```python
from build123d import *

# Parameters (mm, degrees)
BOSS_EXTRUDE1_DEPTH = 1.5875
FILLET1_R           = 2.54
SKETCH6_OUTSIDE_W   = 130.286
SKETCH6_OUTSIDE_H   = 130.286
SKETCH6_OUTSIDE_W_2 = 99
SKETCH6_OUTSIDE_H_2 = 100
CUT_EXTRUDE2_DEPTH  = 71.728496069
SKETCH7_R           = 38.5
BOSS_EXTRUDE2_DEPTH = 0.1


with BuildPart() as part:
    # Sketch1 → Boss-Extrude1 (new body)
    with BuildSketch(Plane.XY):
        Polygon((40, 50), (-40, 50), (-40, 48), (-48, 48), (-48, 40), (-50, 40), (-50, -37.864895224), (-50, -40), (-48, -40), (-48, -48), (-40, -48), (-40, -50), (-37.864895224, -50), (40, -50), (40, -48), (48, -48), (48, -40), (50, -40), (50, 40), (48, 40), (48, 48), (40, 48), align=None)
    extrude(amount=BOSS_EXTRUDE1_DEPTH)

    # Fillet1
    # the kernel refuses this fillet: 2.54 mm, written as the material it adds along each edge
    with BuildSketch(Plane(origin=(-48, -40, 0), x_dir=(0, -1, 0), z_dir=(0, 0, 1)), Plane(origin=(40, -48, 0), x_dir=(1, 0, 0), z_dir=(0, 0, 1)), Plane(origin=(48, 40, 0), x_dir=(0, 1, 0), z_dir=(0, 0, 1)), Plane(origin=(-40, 48, 0), x_dir=(-1, 0, 0), z_dir=(0, 0, 1))) as fillet1_piece_1:
        with BuildLine():
            CenterArc((2.481934729, -2.54), FILLET1_R, 90, 77.725329785)
            Line((0, -2), (-0.049638695, -1.9892))
            ThreePointArc((-0.049638695, -1.9892), (-0.0508, -1), (-0.0508, 0))
            Line((-0.0508, 0), (0, 0.0508))
            Line((0, 0.0508), (2.481934729, 0.0508))
            Line((2.481934729, 0.0508), (2.481934729, 0))
        make_face()
    extrude(amount=1.5875)
    with BuildSketch(Plane(origin=(-40, -48, 0), x_dir=(-3.737454790095179e-12, -1.0, 0), z_dir=(0, 0, 1)), Plane(origin=(48, -40, 0), x_dir=(1.0, -3.7339020764163554e-12, 0), z_dir=(0, 0, 1)), Plane(origin=(-48, 40, 0), x_dir=(-1.0, 3.737454790095126e-12, 0), z_dir=(0, 0, 1))) as fillet1_piece_2:
        with BuildLine():
            CenterArc((2.54, -2.481934729), FILLET1_R, 102.274670215, 77.725329785)
            Line((0, -2.481934729), (-0.0508, -2.481934729))
            Line((-0.0508, -2.481934729), (-0.0508, 0))
            Line((-0.0508, 0), (0, 0.0508))
            ThreePointArc((0, 0.0508), (1, 0.0508), (1.9892, 0.049638695))
            Line((1.9892, 0.049638695), (2, 0))
        make_face()
    extrude(amount=1.5875)
    with BuildSketch(Plane(origin=(40, 48, 0), x_dir=(1, 0, 0), z_dir=(0, 0, 1))) as fillet1_piece_3:
        with BuildLine():
            CenterArc((2.481934729, 2.54), FILLET1_R, 192.274670215, 77.725329785)
            Line((0, 2), (-0.049638695, 1.9892))
            ThreePointArc((-0.049638695, 1.9892), (-0.0508, 1), (-0.0508, 0))
            Line((-0.0508, 0), (0, -0.0508))
            Line((0, -0.0508), (2.481934729, -0.0508))
            Line((2.481934729, -0.0508), (2.481934729, 0))
        make_face()
    extrude(amount=1.5875)

    # Sketch6 outside → Cut-Extrude2 (cut, through all)
    with BuildSketch(Plane.XY.offset(1.5875)):
        Rectangle(SKETCH6_OUTSIDE_W, SKETCH6_OUTSIDE_H)
        Rectangle(SKETCH6_OUTSIDE_W_2, SKETCH6_OUTSIDE_H_2, mode=Mode.SUBTRACT)
    extrude(amount=-CUT_EXTRUDE2_DEPTH, mode=Mode.SUBTRACT)

    # Sketch7 → Boss-Extrude2 (add)
    with BuildSketch(Plane(origin=(0, 0, 0), x_dir=(-1, 0, 0), z_dir=(0, 0, -1))):
        with Locations(Location((0, 0, 0), (0, 0, 180))):
            Circle(SKETCH7_R)
    extrude(amount=BOSS_EXTRUDE2_DEPTH)


solid = part.part
```
The model under review builds one solid part; all positions refer to its coordinate system, in mm. A direction names the side the tool comes from. Coordinates: 2 decimals unless noted, no trailing zeros. Write each loop counter-clockwise with the first axis right and the second up, starting at its lowest first coordinate (ties: lowest second). Pieces come first, ordered by that corner, then holes. Notation, with made-up numbers: (-6.75, -31.5) - (10.25, -31.5) arc R13 ccw to (10.25, -26.5) - close; hole circle Ø2 at (40, 41). An arc over 180 degrees is marked (long way). Answer in a Markdown table with one row per item. Add a question column.
Q1. Consider section B-B on x = -13. Give the boundary of the cut face in (y, z), then the cut area to 3 significant figures.
Q2. Consider section A-A on y = -31.5. Give the boundary of the cut face in (x, z).
Q3. For faces 1 (the face through (-32, 23, 0)), 2 (the face through (-1, -1, -0.1)), list the 3-axis set-ups (+Z, -Z, +X, -X, +Y, -Y) from which the entire face can be reached by the end or side of a thin tool; tool diameter is ignored.
Q4. Clearance check with flat-ended pins moving along their axes: pin 1 (3 mm diameter, centred on x = -34.5, y = 28.5, fed in from -Z); pin 2 (0.8 mm diameter, centred on y = 45.5, z = 0.5, fed in from +X); pin 3 (0.8 mm diameter, centred on x = -45, z = 0.5, fed in from +Y). State where each tip first meets the part, or that it passes through.
Q5. To check wall thickness, follow line 1 along Z through (x, y) = (25.5, 30.5); line 2 along X through (y, z) = (-44.5, 1.3). State the ranges of each line that lie inside material, in increasing order. Write a range as from..to.
Answers below:
| question | item | result |
|---|---|---|
| 1 | outline | (-50, 0) - (-36.24, 0) - (-36.24, -0.1) - (36.24, -0.1) - (36.24, 0) - (50, 0) - (50, 1.59) - (-50, 1.59) - close |
| 1 | area | 166 mm² |
| 2 | outline | (-49.5, 0) - (-22.14, 0) - (-22.14, -0.1) - (22.14, -0.1) - (22.14, 0) - (49.5, 0) - (49.5, 1.59) - (-49.5, 1.59) - close |
| 3 | face 1 | -Z |
| 3 | face 2 | -Z, +X, -X, +Y, -Y |
| 4 | pin 1 | z = 0 |
| 4 | pin 2 | x = 48 |
| 4 | pin 3 | y = 48 |
| 5 | line 1 | 0..1.59 |
| 5 | line 2 | -48..48 |
